```python
from build123d import *

# Parameters (mm, degrees)
BOSS_EXTRUDE2_DEPTH = 11.25
SKETCH3_R           = 1.75
CUT_EXTRUDE1_DEPTH  = 15
SKETCH4_R           = 4.5
CUT_EXTRUDE2_DEPTH  = 5.5


with BuildPart() as part:
    # Sketch2 → Boss-Extrude2 (new body)
    with BuildSketch(Plane(origin=(0, 0, 0), x_dir=(1, 0, 0), z_dir=(0, 1, 0))):
        with BuildLine():
            Line((4.999419692, -0.076175713), (21.999868119, -0.076175713))
            Line((21.999868119, -0.076175713), (21.999868119, -9.076175713))
            Line((21.999868119, -9.076175713), (8.594942375, -9.076175713))
            ThreePointArc((8.594942375, -9.076175713), (0, -12.5), (-8.594942375, -9.076175713))
            Line((-8.594942375, -9.076175713), (-21.999868119, -9.076175713))
            Line((-21.999868119, -9.076175713), (-21.999868119, -0.076175713))
            Line((-21.999868119, -0.076175713), (-4.999419692, -0.076175713))
            ThreePointArc((-4.999419692, -0.076175713), (0, -5), (4.999419692, -0.076175713))
        make_face()
    extrude(amount=BOSS_EXTRUDE2_DEPTH)

    # Sketch3 → Cut-Extrude1 (cut)
    with BuildSketch(Plane.XY.offset(9.076175713)):
        with Locations((15, 5.625)):
            Circle(SKETCH3_R)
        with Locations((-15, 5.625)):
            Circle(SKETCH3_R)
    extrude(amount=-CUT_EXTRUDE1_DEPTH, mode=Mode.SUBTRACT)

    # Sketch4 → Cut-Extrude2 (cut)
    with BuildSketch(Plane.XY.offset(9.076175713)):
        with Locations((15, 5.625)):
            Circle(SKETCH4_R)
        with Locations((-15, 5.625)):
            Circle(SKETCH4_R)
    extrude(amount=-CUT_EXTRUDE2_DEPTH, mode=Mode.SUBTRACT)


solid = part.part
```
Work out the finished part from the listing and answer in its coordinate system (mm). A direction names the side the tool comes from. Round coordinates to 2 decimals unless told otherwise and drop trailing zeros. Loops run counter-clockwise (first coordinate to the right, second up) from the corner with the lowest first, then second, coordinate; pieces in that order, holes last. Notation, with made-up numbers: (38.25, -13.75) -> (71.25, -13.75) arc R29 ccw to (71.25, 14.25) -> close; hole circle Ø2 at (77, -22.75). An arc over 180 degrees is marked (long way). Write each question's results on one line, items separated by ' | '. Start each with the question number.
1. Section B-B (z = 2.5) is taken. Determine the outline of the cut face in (x, y) (3 decimals).
2. For a pull along Y with two mould halves and no side action, classify faces 1 (the face through (0, 0, 6)), 2 (the face through (20, 6, 9.076)), 3 (the face through (-13, 6, 3.576)) as +Y half, -Y half, draft (parallel to the pull), parting line (faces both ways), or undercut.
3. Given pin 1 Ø4.5 at (x, y) = (15, 5.625) entering from -Z; pin 2 Ø4.5 at (x, y) = (17, 5) entering from +Z; pin 3 Ø5.5 at (x, y) = (13, 7) entering from +Z; pin 4 Ø4 at (x, y) = (10.5, 3) entering from +Z, each flat-ended and moving along its own axis, determine where each tip first touches the part or whether it passes through.
4. A tool of negligible diameter and unlimited length cuts with its end or side. For faces 4 (the face through (-20, 6, 9.076)), 5 (the face through (-18.571, 2.887, 6.365)), 6 (the face through (13, 4, 0.076)), from which of +Z, -Z, +X, -X, +Y, -Y can it reach the whole face along a straight path? Write none if from no direction.
5. Section D-D (z = 7) is taken. Determine the outline of the cut face in (x, y) (3 decimals).
6. Section C-C (y = 6.5) is taken. Determine the outline of the cut face in (x, z).
7. Find the intervals of material crossed by probe 1 along Y at (x, z) = (15, 2.05) (3 decimals); probe 2 along X at (y, z) = (8.25, 9); probe 3 along X at (y, z) = (2.75, 8.75), in increasing order. Write a range as from..to.
8. Section A-A (x = -15) is taken. Determine the outline of the cut face in (y, z) (3 decimals).
Evaluation:
1) outline: (-22, 0) -> (-4.33, 0) -> (-4.33, 11.25) -> (-22, 11.25) -> close; (4.33, 0) -> (22, 0) -> (22, 11.25) -> (4.33, 11.25) -> close; hole circle Ø3.5 at (-15, 5.625); hole circle Ø3.5 at (15, 5.625)
2) face 1: -Y half | face 2: draft | face 3: undercut
3) pin 1: stops at z = 0.08 | pin 2: stops at z = 3.58 | pin 3: stops at z = 9.08 | pin 4: stops at z = 9.17
4) face 4: +Z, -X, +Y, -Y | face 5: +Z | face 6: -Z, +X, -X, +Y, -Y
5) outline: (-22, 0) -> (22, 0) -> (22, 11.25) -> (-22, 11.25) -> close; hole circle Ø9 at (-15, 5.625); hole circle Ø9 at (15, 5.625)
6) outline: (-22, 0.08) -> (-16.52, 0.08) -> (-16.52, 3.58) -> (-19.41, 3.58) -> (-19.41, 9.08) -> (-22, 9.08) -> close; (-13.48, 0.08) -> (-5, 0.08) arc R5 cw to (5, 0.08) -> (13.48, 0.08) -> (13.48, 3.58) -> (10.59, 3.58) -> (10.59, 9.08) -> (8.59, 9.08) arc R12.5 ccw to (-8.59, 9.08) -> (-10.59, 9.08) -> (-10.59, 3.58) -> (-13.48, 3.58) -> close; (16.52, 0.08) -> (22, 0.08) -> (22, 9.08) -> (19.41, 9.08) -> (19.41, 3.58) -> (16.52, 3.58) -> close
7) probe 1: y = 0..3.875, 7.375..11.25 | probe 2: x = -22..-18.66, -11.34..11.34, 18.66..22 | probe 3: x = -22..-18.46, -11.54..11.54, 18.46..22
8) outline: (0, 0.076) -> (3.875, 0.076) -> (3.875, 3.576) -> (1.125, 3.576) -> (1.125, 9.076) -> (0, 9.076) -> close; (7.375, 0.076) -> (11.25, 0.076) -> (11.25, 9.076) -> (10.125, 9.076) -> (10.125, 3.576) -> (7.375, 3.576) -> close
